Verification items for the finished model (mm, model axes). A direction names the side the tool comes from. Give positions to 0.01 mm unless a question says otherwise; leave off trailing zeros. Loops run counter-clockwise (first coordinate to the right, second up) from the corner with the lowest first, then second, coordinate; pieces in that order, holes last. Notation, with made-up numbers: M -4,49.25 L 4,49.25 A33 cw 4,80.25 Z; hole C 38,13.5 d7. An arc over 180 degrees is marked long. Use a Markdown table: item, result.
Autodesk Inventor part; units mm, degrees
ref_plane "YZ Plane" through (0, 0, 0) normal (1, 0, 0) x (0, 1, 0)
ref_plane "XZ Plane" through (0, 0, 0) normal (0, 1, 0) x (-1, 0, 0)
ref_plane "XY Plane" through (0, 0, 0) normal (0, 0, 1) x (1, 0, 0)
sketch "Sketch1" plane through (0, 0, 0) normal (1, 0, 0) x (0, 1, 0)
  line L0 (-22, -22) -> (22, -22)
  line L1 (22, -22) -> (22, 22)
  line L2 (22, 22) -> (-22, 22)
  line L3 (-22, 22) -> (-22, -22)
  line L4 (-22, -22) -> (22, 22) construction
  line L5 (22, -22) -> (-22, 22) construction
  line L6 (-19.3, -19.3) -> (19.3, -19.3)
  line L7 (19.3, -19.3) -> (19.3, 19.3)
  line L8 (19.3, 19.3) -> (-19.3, 19.3)
  line L9 (-19.3, 19.3) -> (-19.3, -19.3)
  line L10 (-19.3, -19.3) -> (19.3, 19.3) construction
  line L11 (19.3, -19.3) -> (-19.3, 19.3) construction
  circle A0 centre (19.3, 19.3) radius 1.75
  circle A1 centre (19.3, -19.3) radius 1.75
  circle A2 centre (-19.3, -19.3) radius 1.75
  circle A3 centre (-19.3, 19.3) radius 1.75
  line L12 (19.3, 0) -> (0, 0)
  circle A4 centre (9.5, -9.5) radius 5
  circle A5 centre (9.5, 9.5) radius 5
  line L13 (0, 0) -> (-19.3, 0)
  circle A6 centre (-9.5, -9.5) radius 5
  circle A7 centre (-9.5, 9.5) radius 5
  circle A8 centre (9.5, -9.5) radius 9.5
  circle A9 centre (9.5, 9.5) radius 9.5
  circle A10 centre (-9.5, 9.5) radius 9.5
  circle A11 centre (-9.5, -9.5) radius 9.5
  point P0 (0, 0)
  point P1 (0, 0)
  point P2 (6.364, 6.364)
  dimension "d0" = 44
  dimension "d1" = 44
  dimension "d6" = 38.6
  dimension "d7" = 38.6
  dimension "d8" = 3.5
  dimension "d9" = 3.5
  dimension "d10" = 3.5
  dimension "d11" = 3.5
  dimension "d19" = 10
  dimension "d20" = 10
  dimension "d21" = 10
  dimension "d22" = 10
  dimension "d23" = 19
  dimension "d24" = 19
  dimension "d25" = 19
  dimension "d26" = 19
extrude "Extrusion1" add sketch "Sketch1" along normal blind 2 contours L3 L2 L1 L0 | A2 L9 L13 A11 A8 L12 L7 A1 L6 | L9 A3 L8 A0 L7 L12 A9 A10 L13 | A10 A9 L12 L13 | A10 | L13 L12 A8 A11 | A11 | A9 | A8
fillet "Fillet1" radius 2 4 edges at (1, -22, 22) (1, -22, -22) (1, 22, -22) (1, 22, 22)
sketch "Sketch2" plane through (2, 0, 0) normal (1, 0, 0) x (0, 0, -1)
  arc A0 (-20, 22) -> (-22, 20) centre (-20, 20) ccw
  line L0 (-22, 20) -> (-22, -20)
  arc A1 (-22, -20) -> (-20, -22) centre (-20, -20) ccw
  line L1 (-20, -22) -> (20, -22)
  arc A2 (20, -22) -> (22, -20) centre (20, -20) ccw
  line L2 (22, -20) -> (22, 20)
  arc A3 (22, 20) -> (20, 22) centre (20, 20) ccw
  line L3 (20, 22) -> (-20, 22)
  circle A4 centre (-19.3, -19.3) radius 1.75
  circle A5 centre (19.3, -19.3) radius 1.75
  circle A6 centre (9.5, 9.5) radius 5
  circle A7 centre (9.5, -9.5) radius 5
  circle A8 centre (19.3, 19.3) radius 1.75
  circle A9 centre (-9.5, 9.5) radius 5
  circle A10 centre (-9.5, -9.5) radius 5
  circle A11 centre (-19.3, 19.3) radius 1.75
  circle A12 centre (-9.5, -9.5) radius 8
  circle A13 centre (-9.5, 9.5) radius 8
  circle A14 centre (9.5, 9.5) radius 8
  circle A15 centre (9.5, -9.5) radius 8
  point P0 (0, 0)
  dimension "d27" = 16
  dimension "d28" = 16
  dimension "d29" = 16
  dimension "d30" = 16
extrude "Extrusion2" add sketch "Sketch2" along normal blind 2 contours A12 | A13 | A14 | A15
properties part number "BatteryRoof" material "ABS Plastic"
(1) Cross-section at D-D on z = 9.5. Record the cut outline in (x, y).
Results below:
| item | result |
|---|---|
| outline | M 0,-22 L 2,-22 L 2,-17.5 L 4,-17.5 L 4,-14.5 L 0,-14.5 Z; M 0,-4.5 L 4,-4.5 L 4,-1.5 L 2,-1.5 L 2,1.5 L 4,1.5 L 4,4.5 L 0,4.5 Z; M 0,14.5 L 4,14.5 L 4,17.5 L 2,17.5 L 2,22 L 0,22 Z |
(2) Cross-section at B-B on z = -19.3. Record the cut outline in (x, y).
Results below:
| item | result |
|---|---|
| outline | M 0,-22 L 2,-22 L 2,-21.05 L 0,-21.05 Z; M 0,-17.55 L 2,-17.55 L 2,17.55 L 0,17.55 Z; M 0,21.05 L 2,21.05 L 2,22 L 0,22 Z |
(3) Gauge pin test, flat ends, axial feed: P1, Ø2, axis at y = -9, z = 14, coming from the +X side; P2, Ø2, axis at y = 15.5, z = -2.5, coming from the +X side. Record the tip position at first contact, or that the pin passes through.
Results below:
| item | result |
|---|---|
| P1 | x = 4 |
| P2 | x = 2 |
(4) Cross-section at A-A on x = 3.1. Record the cut outline in (y, z).
Results below:
| item | result |
|---|---|
| outline | C -9.5,-9.5 d16; C -9.5,9.5 d16; C 9.5,-9.5 d16; C 9.5,9.5 d16; hole C -9.5,-9.5 d10; hole C -9.5,9.5 d10; hole C 9.5,-9.5 d10; hole C 9.5,9.5 d10 |
(5) Set-up check for faces 1 (the cylindrical face through (1.01, -21.43, -21.4)), 2 (the flat face through (2, 0, 0)): record each of +Z, -Z, +X, -X, +Y, -Y from which the full face is reachable in a straight line by a thin tool's end or side.
Results below:
| item | result |
|---|---|
| face 1 | -Z, +X, -X, -Y |
| face 2 | +X |
(6) Material ranges on line 1 (Y direction, x = 1.2, z = -9.5); line 2 (Y direction, x = 1.6, z = 19.3), recorded low to high.
Results below:
| item | result |
|---|---|
| line 1 | -22 to -14.5, -4.5 to 4.5, 14.5 to 22 |
| line 2 | -22 to -21.05, -17.55 to 17.55, 21.05 to 22 |
(7) Draft check along Z on faces 3 (the cylindrical face through (2.99, 17.31, 11.23)), 4 (the cylindrical face through (1.01, 21.4, -21.43)), 5 (the cylindrical face through (1.97, 14.14, -11.36)), 6 (the flat face through (1, 22, 0)). Enter one of: +Z half, -Z half, draft (parallel to the pull), parting line (faces both ways), or undercut.
Results below:
| item | result |
|---|---|
| face 3 | undercut |
| face 4 | -Z half |
| face 5 | undercut |
| face 6 | draft |
